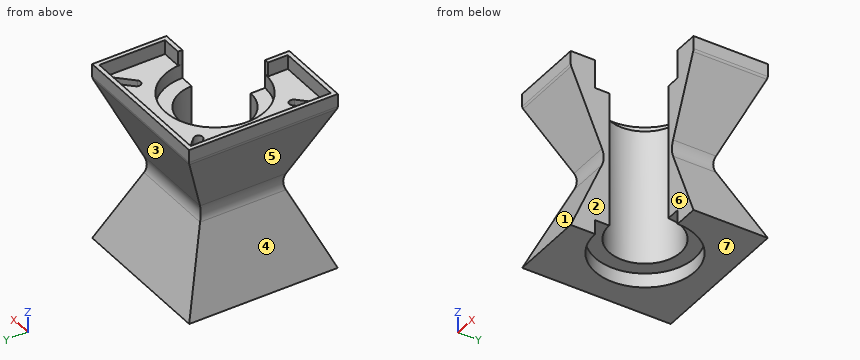
```python
from build123d import *

# Parameters (mm, degrees)
SKETCH1_W           = 104
SKETCH1_H           = 104
BOSS_EXTRUDE1_DEPTH = 57.5
BOSS_EXTRUDE1_TAPER = 23
SKETCH2_R           = 25
CUT_EXTRUDE1_DEPTH  = 137.502747225
SKETCH3_R           = 35
CUT_EXTRUDE2_DEPTH  = 10
CUT_EXTRUDE3_START  = -10
SKETCH4_R           = 35
CUT_EXTRUDE3_DEPTH  = 10
FILLET1_R           = 15
SKETCH6_W           = 52
SKETCH6_H           = 52
CUT_EXTRUDE4_DEPTH  = 137.502747225
BOSS_EXTRUDE2_DEPTH = 10
CUT_EXTRUDE5_DEPTH  = 10
FILLET2_R           = 5


with BuildPart() as part:
    # Sketch1 → Boss-Extrude1 (new body)
    with BuildSketch(Plane.XY):
        Rectangle(SKETCH1_W, SKETCH1_H)
    extrude(amount=BOSS_EXTRUDE1_DEPTH, taper=BOSS_EXTRUDE1_TAPER)

    # Mirror13: part across plane


with BuildPart() as part_1:
    add(part.part)
    add(part.part.mirror(Plane(origin=(0, 0, 57.5), x_dir=(1, 0, 0), z_dir=(0, 0, -1))))

    # Sketch2 → Cut-Extrude1 (cut, through all)
    with BuildSketch(Plane.XY.offset(115)):
        Circle(SKETCH2_R)
    extrude(amount=-CUT_EXTRUDE1_DEPTH, mode=Mode.SUBTRACT)

    # Sketch3 → Cut-Extrude2 (cut)
    with BuildSketch(Plane.XY.offset(115)):
        Circle(SKETCH3_R)
    extrude(amount=-CUT_EXTRUDE2_DEPTH, mode=Mode.SUBTRACT)

    # Sketch4 → Cut-Extrude3 (cut)
    with BuildSketch(Plane(origin=(0, 0, 0), x_dir=(-1, 0, 0), z_dir=(0, 0, -1)).offset(CUT_EXTRUDE3_START)):
        with Locations(Location((0, 0, 0), (0, 0, 180))):
            Circle(SKETCH4_R)
    extrude(amount=CUT_EXTRUDE3_DEPTH, mode=Mode.SUBTRACT)

    # Fillet1
    fillet1_edges = [part_1.edges().sort_by_distance(p)[0] for p in [
        (27.592698068, 0, 57.5),
        (0, 27.592698068, 57.5),
        (-27.592698068, 0, 57.5),
        (0, -27.592698068, 57.5),
    ]]
    fillet(fillet1_edges, radius=FILLET1_R)

    # Sketch6 → Cut-Extrude4 (cut, through all)
    with BuildSketch(Plane.XY.offset(115)):
        with Locations((26, -26)):
            Rectangle(SKETCH6_W, SKETCH6_H)
    extrude(amount=-CUT_EXTRUDE4_DEPTH, mode=Mode.SUBTRACT)

    # Sketch7 → Boss-Extrude2 (add)
    with BuildSketch(Plane.XY.offset(115)):
        Polygon((49, 49), (49, 3), (35, 3), (35, 0), (52, 0), (52, 52), (-52, 52), (-52, -52), (0, -52), (0, -35), (-3, -35), (-3, -49), (-49, -49), (-49, 49), align=None)
    extrude(amount=BOSS_EXTRUDE2_DEPTH)

    # Sketch8 → Cut-Extrude5 (cut)
    with BuildSketch(Plane.XY.offset(115)):
        with BuildLine():
            Line((-41.805559998, 46.048200685), (-31.19895828, 35.441598967))
            ThreePointArc((-31.19895828, 35.441598967), (-31.19895828, 31.19895828), (-35.441598967, 31.19895828))
            Line((-35.441598967, 31.19895828), (-46.048200685, 41.805559998))
            ThreePointArc((-46.048200685, 41.805559998), (-46.048200685, 46.048200685), (-41.805559998, 46.048200685))
        make_face()
        with BuildLine():
            Line((46.048200685, 41.805559998), (35.441598967, 31.19895828))
            ThreePointArc((35.441598967, 31.19895828), (31.19895828, 31.19895828), (31.19895828, 35.441598967))
            Line((31.19895828, 35.441598967), (41.805559998, 46.048200685))
            ThreePointArc((41.805559998, 46.048200685), (46.048200685, 46.048200685), (46.048200685, 41.805559998))
        make_face()
        with BuildLine():
            Line((-46.048200685, -41.805559998), (-35.441598967, -31.19895828))
            ThreePointArc((-35.441598967, -31.19895828), (-31.19895828, -31.19895828), (-31.19895828, -35.441598967))
            Line((-31.19895828, -35.441598967), (-41.805559998, -46.048200685))
            ThreePointArc((-41.805559998, -46.048200685), (-46.048200685, -46.048200685), (-46.048200685, -41.805559998))
        make_face()
    extrude(amount=-CUT_EXTRUDE5_DEPTH, mode=Mode.SUBTRACT)

    # Fillet2
    fillet2_edges = [part_1.edges().sort_by_distance(p)[0] for p in [
        (0, 52, 115),
        (-52, 0, 115),
        (-26, -52, 115),
        (52, 26, 115),
    ]]
    fillet(fillet2_edges, radius=FILLET2_R)


solid = part_1.part
```
Part model, mm, in its own coordinate system. Face numbers are marked on the shaded views. A direction names the side the tool comes from. Round coordinates to 2 decimals unless told otherwise and drop trailing zeros. Loops run counter-clockwise (first coordinate to the right, second up) from the corner with the lowest first, then second, coordinate; pieces in that order, holes last.
1. Slice it at A-A (y = 40). Give the cut face in (x, z), and give its area (3 significant figures).
Solutions:
outline: (-52, 0) - (52, 0) - (40, 28.27) - (-40, 28.27) - close; (-52, 116.02) arc R5 ccw to (-51.6, 114.06) - (-40, 86.73) - (40, 86.73) - (51.6, 114.06) arc R5 ccw to (52, 116.02) - (52, 125) - (49, 125) - (49, 115) - (44.24, 115) - (44.24, 105) - (35.76, 105) - (35.76, 115) - (-35.76, 115) - (-35.76, 105) - (-44.24, 105) - (-44.24, 115) - (-49, 115) - (-49, 125) - (-52, 125) - close
area: 5,090 mm2
2. Slice it at D-D (z = 30). Give the cut face in (x, y), and give its area (3 significant figures).
Solutions:
outline: (-39.27, -39.27) - (0, -39.27) - (0, -25) arc R25 cw (long way) to (25, 0) - (39.27, 0) - (39.27, 39.27) - (-39.27, 39.27) - close
area: 3,150 mm2
3. Flat gauge pins, fed straight in: pin 1 (6 mm diameter, centred on x = -13, y = 24.5, fed in from -Z); pin 2 (10 mm diameter, centred on x = 33, z = 74, fed in from +Y); pin 3 (2 mm diameter, centred on x = 7.5, z = 82.5, fed in from -Y); pin 4 (12 mm diameter, centred on y = 39, z = 49, fed in from -X). Where does each tip first touch, or does it go through?
Solutions:
pin 1: stops at z = 10
pin 2: stops at y = 36.72
pin 3: stops at y = 23.51
pin 4: passes through
4. 3-axis set-ups, long thin cutter, end or side, ignore diameter. For the marked faces 1, 2, 3 and 4: which of +Z, -Z, +X, -X, +Y, -Y reach the whole face in a straight line?
Solutions:
face 1: +X, -X, -Y
face 2: +Z, -Z, +X, -Y
face 3: +X, -X, +Y
face 4: -X, +Y, -Y
5. Drill centre lines: line 1 along Z through (x, y) = (30.5, 11); line 2 along Z through (x, y) = (42, 28.5); line 3 along Y through (x, z) = (-28, 12). Where is each one in solid material? Low to high.
Solutions:
line 1: z = 10 to 50.65, 64.35 to 105
line 2: z = 0 to 23.56, 91.44 to 115
line 3: y = -46.91 to 46.91
6. Slice it at C-C (x = 21.5). Give the cut face in (y, z), and give its area (3 significant figures).
Solutions:
outline: (12.76, 10) - (27.62, 10) - (27.62, 0) - (52, 0) - (30.08, 51.64) arc R15 cw to (30.08, 63.36) - (51.6, 114.06) arc R5 ccw to (52, 116.02) - (52, 125) - (49, 125) - (49, 115) - (27.62, 115) - (27.62, 105) - (12.76, 105) - close
area: 2,850 mm2
7. Two-plate mould, pull along Z, no slides. Class the marked faces 5, 6 and 7: pulls with the +Z half, pulls with the -Z half, needs draft (parallel to the pull), parting line crosses it, or undercut.
Solutions:
face 5: undercut
face 6: needs draft
face 7: pulls with the -Z half
8. Slice it at B-B (z = 94). Give the cut face in (x, y), and give its area (3 significant figures).
Solutions:
outline: (-43.09, -43.09) - (0, -43.09) - (0, -25) arc R25 cw (long way) to (25, 0) - (43.09, 0) - (43.09, 43.09) - (-43.09, 43.09) - close
area: 4,100 mm2
